```python
from build123d import *

# Parameters (mm, degrees)
F3_D = 22.225
F5_D = 6.35


with BuildPart() as f1:
    # F0 (on Front) → F1 (revolve)
    with BuildSketch(Plane.XZ):
        Polygon((0, 31.75), (0, 0), (35.615216, 0), (35.615216, 6.35), (12.7, 6.35), (12.7, 31.75), align=None)
    revolve(axis=Axis((0, 0, 15.875), (0, 0, -1)))

    # F3 (through all)
    with Locations(Plane.XY.offset(31.75)):
        with Locations((0, 0)):
            Hole(F3_D / 2)

    # F5 (through all)
    with Locations(Plane.XY.offset(6.35)):
        with Locations((0, 25.39767)):
            Hole(F5_D / 2)


solid = f1.part
```
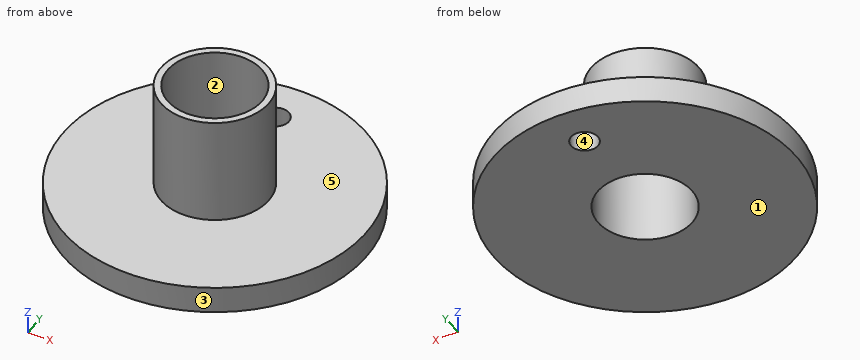
Design review of the part built by this model. Coordinates are the model's own, in mm. Face numbers are marked on the shaded views. A direction names the side the tool comes from. Coordinates: 2 decimals unless noted, no trailing zeros. Order: outer loops, then holes, each group sorted by start corner. A loop starts at its lowest first (then second) coordinate and runs counter-clockwise, first axis right, second up. Notation, with made-up numbers: (60, 36.25) -> (97, 36.25) arc R22 cw to (97, 46.25) -> close; hole circle Ø7 at (18, -23). An arc over 180 degrees is marked (long way). One line per item, written item: value. Start each with the question number.
Q1. For probe 1 along Y at (x, z) = (0, 5); probe 2 along Y at (x, z) = (0, 12); probe 3 along Z at (x, y) = (-15.5, -15), list the stretches that pass through material, from the lowest coordinate up.
Q2. Take a section at D-D, the plane z = 28. State the section outline as (x, y) points (1 decimal), then the cut area to 3 significant figures.
Q3. Insertion check: pin 1 Ø4 at (y, z) = (1, 26.5) entering from +X; pin 2 Ø3 at (y, z) = (-27.5, 3.5) entering from +X; pin 3 Ø4 at (y, z) = (6, 19) entering from +X. Each pin has a flat end and moves straight along its axis. Give the tip position at first contact, or say it passes through.
Q4. Take a section at C-C, the plane y = 24.5. State the section outline as (x, z) points.
Q5. Tool access review of the marked faces 4 and 5: name each direction out of +Z, -Z, +X, -X, +Y, -Y from which nothing blocks a thin tool from reaching the whole face with its end or side.
Q6. Take a section at B-B, the plane y = 0. State the section outline as (x, z) points.
Q7. Take a section at A-A, the plane x = 0. State the section outline as (y, z) points, then the cut area to 3 significant figures.
Q8. Mouldability with a two-part tool opening along X and no side actions: class the marked faces 1, 2 and 3 as pulls with the +X half, pulls with the -X half, needs draft (parallel to the pull), parting line crosses it, or undercut.
Values follow:
1. probe 1: y = -35.62 to -11.11, 11.11 to 22.22, 28.57 to 35.62
1. probe 2: y = -12.7 to -11.11, 11.11 to 12.7
1. probe 3: z = 0 to 6.35
2. outline: circle Ø25.4 at (0, 0); hole circle Ø22.2 at (0, 0)
2. area: 119 mm2
3. pin 1: stops at x = 12.7
3. pin 2: stops at x = 24.34
3. pin 3: stops at x = 12.05
4. outline: (-25.85, 0) -> (-3.05, 0) -> (-3.05, 6.35) -> (-25.85, 6.35) -> close; (3.05, 0) -> (25.85, 0) -> (25.85, 6.35) -> (3.05, 6.35) -> close
5. face 4: +Z, -Z
5. face 5: +Z
6. outline: (-35.62, 0) -> (-11.11, 0) -> (-11.11, 31.75) -> (-12.7, 31.75) -> (-12.7, 6.35) -> (-35.62, 6.35) -> close; (11.11, 0) -> (35.62, 0) -> (35.62, 6.35) -> (12.7, 6.35) -> (12.7, 31.75) -> (11.11, 31.75) -> close
7. outline: (-35.62, 0) -> (-11.11, 0) -> (-11.11, 31.75) -> (-12.7, 31.75) -> (-12.7, 6.35) -> (-35.62, 6.35) -> close; (11.11, 0) -> (22.22, 0) -> (22.22, 6.35) -> (12.7, 6.35) -> (12.7, 31.75) -> (11.11, 31.75) -> close; (28.57, 0) -> (35.62, 0) -> (35.62, 6.35) -> (28.57, 6.35) -> close
7. area: 352 mm2
8. face 1: needs draft
8. face 2: undercut
8. face 3: parting line crosses it
